Build history of the part. All positions in model axes, mm. Give positions to 0.01 mm unless a question says otherwise; leave off trailing zeros. Order: outer loops, then holes, each group sorted by start corner. A loop starts at its lowest first (then second) coordinate and runs counter-clockwise, first axis right, second up. Notation, with made-up numbers: M 57.5,63 L 72.5,63 A8 cw 72.5,69 Z; hole C 56,69.5 d5. An arc over 180 degrees is marked long. One line per item, written item: value.
from build123d import *

# Parameters (mm, degrees)
SKETCH2_W           = 80
SKETCH2_H           = 12.7
BOSS_EXTRUDE1_DEPTH = 12.7
SKETCH3_R           = 2
SKETCH3_R_2         = 2.5
CUT_EXTRUDE1_DEPTH  = 43.445406112
SKETCH4_RX          = 8.89
SKETCH4_RY          = 4.6609
CUT_EXTRUDE3_DEPTH  = 44.847234804


with BuildPart() as part:
    # Sketch2 → Boss-Extrude1 (new body)
    with BuildSketch(Plane(origin=(0, 0, 0), x_dir=(1, 0, 0), z_dir=(0, 1, 0))):
        Rectangle(SKETCH2_W, SKETCH2_H)
    extrude(amount=BOSS_EXTRUDE1_DEPTH)

    # Sketch3 → Cut-Extrude1 (cut, through all)
    with BuildSketch(Plane(origin=(0, 12.7, 0), x_dir=(1, 0, 0), z_dir=(0, 1, 0))):
        with Locations(Location((-35, 0, 0), (0, 0, 270))):
            Circle(SKETCH3_R)
        with Locations(Location((-20, 0, 0), (0, 0, 270))):
            Circle(SKETCH3_R)
        with Locations(Location((35, 0, 0), (0, 0, 270))):
            Circle(SKETCH3_R_2)
        with Locations(Location((20, 0, 0), (0, 0, 270))):
            Circle(SKETCH3_R_2)
    extrude(amount=-CUT_EXTRUDE1_DEPTH, mode=Mode.SUBTRACT)

    # Sketch4 → Cut-Extrude3 (cut, through all)
    with BuildSketch(Plane.XY.offset(6.35)):
        with Locations((0, 6.20775407)):
            Ellipse(SKETCH4_RX, SKETCH4_RY)
    extrude(amount=-CUT_EXTRUDE3_DEPTH, mode=Mode.SUBTRACT)


solid = part.part
1) Saw through at B-B, the plane z = 0.5. Give the number of separate pieces and of enclosed holes in the cut face, then the cut area to 3 significant figures.
Check values:
separate pieces: 5
enclosed holes: 1
area: 663 mm^2
2) Saw through at A-A, the plane x = -35. Write the cut outline in (y, z), then the cut area to 3 significant figures.
Check values:
outline: M 0,-6.35 L 12.7,-6.35 L 12.7,-2 L 0,-2 Z; M 0,2 L 12.7,2 L 12.7,6.35 L 0,6.35 Z
area: 110 mm^2
3) Drill centre lines: probe 1 along X at (y, z) = (7, 0); probe 2 along X at (y, z) = (3, 0); probe 3 along Y at (x, z) = (6.5, 3.5). Where is each one in solid material? Low to high. Write a range as from..to.
Check values:
probe 1: -40..-37, -33..-22, -18..-8.76, 8.76..17.5, 22.5..32.5, 37.5..40
probe 2: -40..-37, -33..-22, -18..-6.45, 6.45..17.5, 22.5..32.5, 37.5..40
probe 3: 0..3.03, 9.39..12.7
4) Saw through at D-D, the plane x = 20. Write the cut outline in (y, z).
Check values:
outline: M 0,-6.35 L 12.7,-6.35 L 12.7,-2.5 L 0,-2.5 Z; M 0,2.5 L 12.7,2.5 L 12.7,6.35 L 0,6.35 Z
5) Mould opens along X. For faces 1 (the face through (-1, 12, -6.35)), 2 (the face through (40, 6, 0)), 3 (the face through (-37, 6, 0)) say: released by +X, released by -X, zero draft, split by the parting line, or undercut.
Check values:
face 1: zero draft
face 2: released by +X
face 3: undercut
6) Pin check, flat tip, straight feed: pin 1 (3 mm diameter, centred on x = 35, z = 0, fed in from -Y). Stop position of the tip, or through.
Check values:
pin 1: through
